CAD build for the part. Positions are in the model's coordinates, mm. Coordinates: 2 decimals unless noted, no trailing zeros. Loops run counter-clockwise (first coordinate to the right, second up) from the corner with the lowest first, then second, coordinate; pieces in that order, holes last. Notation, with made-up numbers: (10.25, 27) -> (38.25, 27) arc R18 cw to (38.25, 50) -> close; hole circle Ø3 at (80.25, -13.5). An arc over 180 degrees is marked (long way). Return JSON: item names as keys, results as strings. Group by question number.
(1) Saw through at B-B on z = -0.75. Write the cut outline in (x, y).
(2) Flat gauge pins, fed straight in: pin 1 Ø1.5 at (x, y) = (-50.8, 0) entering from -Z; pin 2 Ø1 at (y, z) = (1, 0.5) entering from +X. Where does each tip first touch, or does it go through?
(3) Probe L1, parallel to Y at x = 50.8, z = -0.55; L2, parallel to X at y = -0.9, z = -1.2; L3, parallel to X at y = -0.5, z = -0.35. List the from-to ranges inside material, lowest first.
(4) Saw through at A-A on y = 0. Write the cut outline in (x, z), then the cut area to 3 significant figures.
```python
from build123d import *

# Parameters (mm, degrees)
BOSS_EXTRUDE1_DEPTH      = 1.42
BOSS_EXTRUDE1_DEPTH_BACK = 1.42
SKETCH1_R                = 1.27


with BuildPart() as part:
    # Sketch1 → Boss-Extrude1 (new, two sides: drawn at the far end of the back side and taken through both)
    with BuildSketch(Plane.XY.offset(-BOSS_EXTRUDE1_DEPTH_BACK)):
        with BuildLine():
            Line((-50.8, 2.54), (50.8, 2.54))
            ThreePointArc((50.8, 2.54), (53.34, 0), (50.8, -2.54))
            Line((50.8, -2.54), (-50.8, -2.54))
            ThreePointArc((-50.8, -2.54), (-53.34, 0), (-50.8, 2.54))
        make_face()
        with Locations((-50.8, 0)):
            Circle(SKETCH1_R, mode=Mode.SUBTRACT)
        with Locations((50.8, 0)):
            Circle(SKETCH1_R, mode=Mode.SUBTRACT)
    extrude(amount=BOSS_EXTRUDE1_DEPTH + BOSS_EXTRUDE1_DEPTH_BACK)


solid = part.part
```
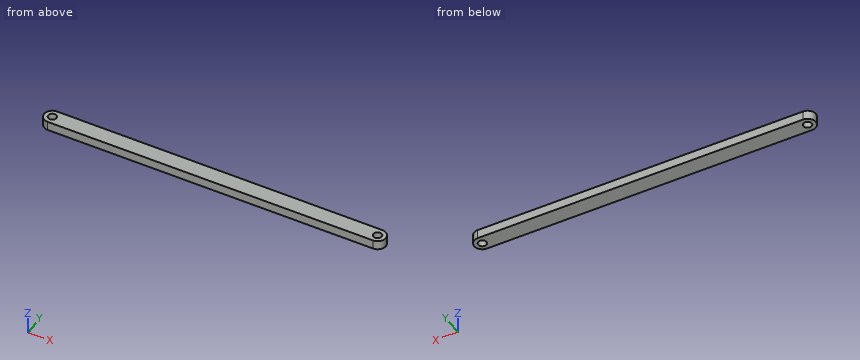
Geometry results:
{
 "1": {"outline": "(-50.8, -2.54) -> (50.8, -2.54) arc R2.54 ccw to (50.8, 2.54) -> (-50.8, 2.54) arc R2.54 ccw to start; hole circle Ø2.54 at (-50.8, 0); hole circle Ø2.54 at (50.8, 0)"},
 "2": {"pin 1": "through", "pin 2": "x = 53.29"},
 "3": {"L1": "-2.54 to -1.27, 1.27 to 2.54", "L2": "-53.18 to -51.7, -49.9 to 49.9, 51.7 to 53.18", "L3": "-53.29 to -51.97, -49.63 to 49.63, 51.97 to 53.29"},
 "4": {"outline": "(-53.34, -1.42) -> (-52.07, -1.42) -> (-52.07, 1.42) -> (-53.34, 1.42) -> close; (-49.53, -1.42) -> (49.53, -1.42) -> (49.53, 1.42) -> (-49.53, 1.42) -> close; (52.07, -1.42) -> (53.34, -1.42) -> (53.34, 1.42) -> (52.07, 1.42) -> close", "area": "289 mm²"}
}
